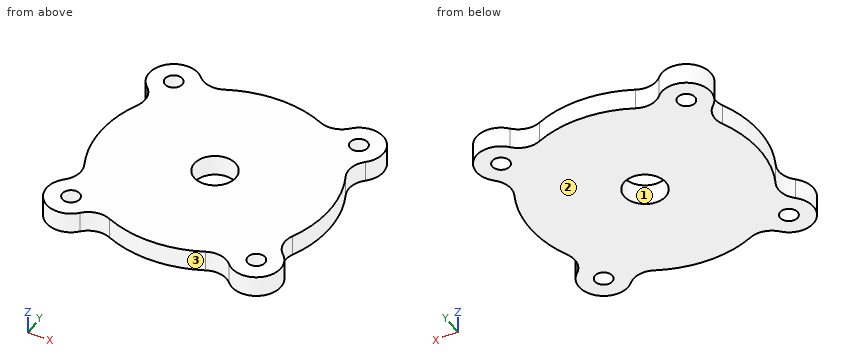
```python
from build123d import *

# Parameters (mm, degrees)
BOSS_EXTRUDE1_DEPTH      = 3.175
FILLET1_R                = 7
M5_CLEARANCE_HOLE1_D     = 5.3
M5_CLEARANCE_HOLE1_DEPTH = 6.35
M5_CLEARANCE_HOLE1_TIP   = 1.59228064
SKETCH4_R                = 6.35
CUT_EXTRUDE1_DEPTH       = 52.003437659


with BuildPart() as part:
    # Sketch1 → Boss-Extrude1 (new, symmetric)
    with BuildSketch(Plane.XY):
        with BuildLine():
            ThreePointArc((-20.785305148, 28.159742362), (-33.587572106, 33.587572106), (-28.159742362, 20.785305148))
            ThreePointArc((-28.159742362, 20.785305148), (-35, 0), (-28.159742362, -20.785305148))
            ThreePointArc((-28.159742362, -20.785305148), (-33.587572106, -33.587572106), (-20.785305148, -28.159742362))
            ThreePointArc((-20.785305148, -28.159742362), (0, -35), (20.785305148, -28.159742362))
            ThreePointArc((20.785305148, -28.159742362), (33.587572106, -33.587572106), (28.159742362, -20.785305148))
            ThreePointArc((28.159742362, -20.785305148), (35, 0), (28.159742362, 20.785305148))
            ThreePointArc((28.159742362, 20.785305148), (33.587572106, 33.587572106), (20.785305148, 28.159742362))
            ThreePointArc((20.785305148, 28.159742362), (0, 35), (-20.785305148, 28.159742362))
        make_face()
    extrude(amount=BOSS_EXTRUDE1_DEPTH, both=True)

    # Fillet1
    fillet1_edges = [part.edges().sort_by_distance(p)[0] for p in [
        (20.785305148, 28.159742362, 0),
        (28.159742362, 20.785305148, 0),
        (28.159742362, -20.785305148, 0),
        (20.785305148, -28.159742362, 0),
        (-20.785305148, -28.159742362, 0),
        (-28.159742362, -20.785305148, 0),
        (-28.159742362, 20.785305148, 0),
        (-20.785305148, 28.159742362, 0),
    ]]
    fillet(fillet1_edges, radius=FILLET1_R)

    # M5 Clearance Hole1
    with Locations(Plane.XY.offset(3.175)):
        with Locations((-28.284271247, 28.284271247), (28.284271247, 28.284271247), (28.284271247, -28.284271247), (-28.284271247, -28.284271247)):
            Hole(M5_CLEARANCE_HOLE1_D / 2, depth=M5_CLEARANCE_HOLE1_DEPTH)
            with Locations((0, 0, -(M5_CLEARANCE_HOLE1_DEPTH + M5_CLEARANCE_HOLE1_TIP / 2))):  # 118° drill point
                Cone(0, M5_CLEARANCE_HOLE1_D / 2, M5_CLEARANCE_HOLE1_TIP, mode=Mode.SUBTRACT)

    # Sketch4 → Cut-Extrude1 (cut, through all)
    with BuildSketch(Plane.XY.offset(3.175)):
        Circle(SKETCH4_R)
    extrude(amount=-CUT_EXTRUDE1_DEPTH, mode=Mode.SUBTRACT)


solid = part.part
```
The model under review builds one solid part; all positions refer to its coordinate system, in mm. Face numbers are marked on the shaded views. Round coordinates to 2 decimals unless told otherwise and drop trailing zeros. Order: outer loops, then holes, each group sorted by start corner. A loop starts at its lowest first (then second) coordinate and runs counter-clockwise, first axis right, second up.
(1) Wall thickness on L1, parallel to X at y = -28, z = -2; L2, parallel to Y at x = 32, z = 1; L3, parallel to X at y = 29.5, z = -1.25: over which ranges is each line inside the solid? List them lowest first.
Working result:
L1: x = -35.78 to -30.92, -25.65 to 25.65, 30.92 to 35.78
L2: y = -34.8 to -21.03, -14.18 to 14.18, 21.03 to 34.8
L3: x = -35.69 to -30.64, -25.93 to 25.93, 30.64 to 35.69
(2) Take a section at A-A, the plane y = 0. State the section outline as (x, z) points (3 decimals), plus the area to 3 significant figures.
Working result:
outline: (-35, -3.175) - (-6.35, -3.175) - (-6.35, 3.175) - (-35, 3.175) - close; (6.35, -3.175) - (35, -3.175) - (35, 3.175) - (6.35, 3.175) - close
area: 364 mm2
(3) For P1, Ø1.5, axis at y = -4, z = -1, coming from the -X side; P2, Ø3, axis at y = 12, z = 0.5, coming from the -X side; P3, Ø1, axis at x = -15.5, z = 2.5, coming from the +Y side, all flat-tipped, find the tip position at first contact; note any pin that passes through.
Working result:
P1: stops at x = -34.85
P2: stops at x = -33.39
P3: stops at y = 31.63
(4) Take a section at D-D, the plane x = 10. State the section outline as (y, z) points (3 decimals), plus the area to 3 significant figures.
Working result:
outline: (-33.541, -3.175) - (33.541, -3.175) - (33.541, 3.175) - (-33.541, 3.175) - close
area: 426 mm2
(5) Take a section at C-C, the plane z = 0.25. Count the separate pieces of the cut face and the enclosed holes in it, plus the area to 3 significant figures.
Working result:
separate pieces: 1
enclosed holes: 5
area: 4,340 mm2
(6) Mouldability with a two-part tool opening along Y and no side actions: class the marked faces 1, 2 and 3 as released by +Y, released by -Y, zero draft, split by the parting line, or undercut.
Working result:
face 1: undercut
face 2: zero draft
face 3: released by -Y
